Could you check a few things on this model? Use its own coordinates, in mm. A direction names the side the tool comes from. Coordinates: 2 decimals unless noted, no trailing zeros. Order: outer loops, then holes, each group sorted by start corner. A loop starts at its lowest first (then second) coordinate and runs counter-clockwise, first axis right, second up. Notation, with made-up numbers: (-26.5, 30) - (21.5, 30) arc R15 ccw to (21.5, 54) - close; hole circle Ø10 at (-13.75, 50.25). An arc over 180 degrees is marked (long way). One line per item, written item: value.
from build123d import *

# Parameters (mm, degrees)
BOSS_EXTRUDE2_DEPTH = 101.6
BOSS_EXTRUDE3_DEPTH = 5.08
SKETCH4_R           = 6.35
CUT_EXTRUDE1_DEPTH  = 156.040615371


with BuildPart() as part:
    # Sketch1 → Boss-Extrude2 (new body)
    with BuildSketch(Plane(origin=(0, 0, 0), x_dir=(1, 0, 0), z_dir=(0, 1, 0))):
        with BuildLine():
            Line((-21.298547486, 13.839504146), (-21.298547486, 45.589504146))
            Line((-21.298547486, 45.589504146), (21.298547486, 45.589504146))
            Line((21.298547486, 45.589504146), (21.298547486, 13.839504146))
            ThreePointArc((21.298547486, 13.839504146), (0, 25.4), (-21.298547486, 13.839504146))
        make_face()
    extrude(amount=BOSS_EXTRUDE2_DEPTH)

    # Sketch3 → Boss-Extrude3 (add)
    with BuildSketch(Plane.ZY.offset(21.298547486)):
        with BuildLine():
            Line((-45.589504146, 63.5), (-96.389504146, 63.5))
            ThreePointArc((-96.389504146, 63.5), (-109.089504146, 50.8), (-96.389504146, 38.1))
            Line((-96.389504146, 38.1), (-45.589504146, 38.1))
            Line((-45.589504146, 38.1), (-45.589504146, 63.5))
        make_face()
    boss_extrude3 = extrude(amount=-BOSS_EXTRUDE3_DEPTH)

    # Sketch4 → Cut-Extrude1 (cut, through all)
    with BuildSketch(Plane.ZY.offset(21.298547486)):
        with Locations((-96.389504146, 50.8)):
            Circle(SKETCH4_R)
    cut_extrude1 = extrude(amount=-CUT_EXTRUDE1_DEPTH, mode=Mode.SUBTRACT)

    # Mirror1: Boss-Extrude3, Cut-Extrude1 across plane
    add(boss_extrude3.mirror(Plane(origin=(0, 0, 0), x_dir=(0, 0, 1), z_dir=(1, 0, 0))))
    add(cut_extrude1.mirror(Plane(origin=(0, 0, 0), x_dir=(0, 0, 1), z_dir=(1, 0, 0))), mode=Mode.SUBTRACT)


solid = part.part
Item 1: I want a section at B-B on y = 50.8. Please give me the cut outline in (x, z).
Conclusion:
outline: (-21.3, -109.09) - (-16.22, -109.09) - (-16.22, -102.74) - (-21.3, -102.74) - close; (-21.3, -90.04) - (-16.22, -90.04) - (-16.22, -45.59) - (16.22, -45.59) - (16.22, -90.04) - (21.3, -90.04) - (21.3, -13.84) arc R25.4 cw to (-21.3, -13.84) - close; (16.22, -109.09) - (21.3, -109.09) - (21.3, -102.74) - (16.22, -102.74) - close
Item 2: I'm going to push flat-ended pins straight in: pin 1 Ø4 at (x, y) = (-5, 18) entering from -Z; pin 2 Ø6 at (x, z) = (-10.5, -70) entering from +Y; pin 3 Ø1 at (x, y) = (-5, 18) entering from +Z; pin 4 Ø5.5 at (x, z) = (17.5, -60.5) entering from +Y. Where does each tip first touch, or does it pass through?
Conclusion:
pin 1: z = -45.59
pin 2: through
pin 3: z = -24.8
pin 4: y = 63.5
Item 3: If I drill on probe 1 along X at (y, z) = (42, -71.5); probe 2 along Y at (x, z) = (16.5, -76); probe 3 along X at (y, z) = (61.5, -22.5), over which ranges is the centre line in solid material (lowest first)?
Conclusion:
probe 1: -21.3 to -16.22, 16.22 to 21.3
probe 2: 38.1 to 63.5
probe 3: -21.3 to -11.79, 11.79 to 21.3
Item 4: I want a section at D-D on y = 95. Please give me the cut outline in (x, z), then the cut area to 3 significant figures.
Conclusion:
outline: (-21.3, -45.59) - (21.3, -45.59) - (21.3, -13.84) arc R25.4 cw to (-21.3, -13.84) - close
area: 1,010 mm²
Item 5: I want a section at A-A on z = -52.5. Please give me the cut outline in (x, y), then the cut area to 3 significant figures.
Conclusion:
outline: (-21.3, 38.1) - (-16.22, 38.1) - (-16.22, 63.5) - (-21.3, 63.5) - close; (16.22, 38.1) - (21.3, 38.1) - (21.3, 63.5) - (16.22, 63.5) - close
area: 258 mm²
Item 6: Thinking about a two-plate mould opening in Y: for faces 1 (the face through (18.794, 56.154, -92.976)), 2 (the face through (-19, 63.5, -71)), 3 (the face through (16.219, 51, -78)), which applies, pulls with the +Y half, pulls with the -Y half, needs draft (parallel to the pull), parting line crosses it, or undercut?
Conclusion:
face 1: undercut
face 2: pulls with the +Y half
face 3: needs draft
Item 7: I want a section at C-C on z = -20. Please give me the cut outline in (x, y).
Conclusion:
outline: (-21.3, 0) - (-15.66, 0) - (-15.66, 101.6) - (-21.3, 101.6) - close; (15.66, 0) - (21.3, 0) - (21.3, 101.6) - (15.66, 101.6) - close
Item 8: For faces 4 (the face through (-18.794, 51.079, -109.086)), 5 (the face through (19, 38.1, -71)), 6 (the face through (-16.219, 51, -78)), 7 (the face through (19, 63.5, -71)), which set-ups out of +Z, -Z, +X, -X, +Y, -Y let a thin tool reach every point of the face, with its end or its side?
Conclusion:
face 4: -Z, +X, -X
face 5: -Z, +X, -X, -Y
face 6: -Z, +Y, -Y
face 7: -Z, +X, -X, +Y
